Read the model definition and answer for the solid it produces. Units are mm, in the model's axes. Face numbers are marked on the shaded views. A direction names the side the tool comes from. Round coordinates to 2 decimals unless told otherwise and drop trailing zeros. Loops run counter-clockwise (first coordinate to the right, second up) from the corner with the lowest first, then second, coordinate; pieces in that order, holes last. Notation, with made-up numbers: M -3,13.5 L 40,13.5 A37 ccw 40,49.5 Z; hole C 46.25,6.25 d6. An arc over 180 degrees is marked long. Write each question's results on one line, items separated by ' | '.
Autodesk Inventor part; units mm, degrees
ref_plane "YZ Plane" through (0, 0, 0) normal (1, 0, 0) x (0, 1, 0)
ref_plane "XZ Plane" through (0, 0, 0) normal (0, 1, 0) x (-1, 0, 0)
ref_plane "XY Plane" through (0, 0, 0) normal (0, 0, 1) x (1, 0, 0)
sketch "Sketch1" plane through (0, 0, 0) normal (0, 0, 1) x (1, 0, 0)
  line L0 (-21, 8) -> (21, 8)
  line L1 (21, 8) -> (21, -21)
  line L2 (21, -21) -> (-21, -21)
  line L3 (-21, -21) -> (-21, 8)
  point P0 (0, 0)
  point P1 (0, -21)
  dimension "d0" = 21
  dimension "d1" = 42
  dimension "d2" = 29
extrude "Extrusion1" add sketch "Sketch1" along normal blind 15
fillet "Fillet1" radius 5 4 edges at (21, -21, 7.5) (-21, 8, 7.5) (21, 8, 7.5) (-21, -21, 7.5)
sketch "Sketch2" plane through (0, 0, 15) normal (0, 0, 1) x (1, 0, 0)
  line L0 (16, 8) -> (-16, 8)
  arc A0 (-11.05, 0) -> (11.05, 0) centre (0, 0) ccw
  line L1 (-11.05, 0) -> (-11.05, 8)
  line L2 (11.05, 0) -> (11.05, 8)
  dimension "d6" = 11.05
extrude "Extrusion2" cut sketch "Sketch2" against normal blind 3
sketch "Sketch3" plane through (0, 0, 12) normal (0, 0, 1) x (1, 0, 0)
  arc A0 (-11.05, 0) -> (11.05, 0) centre (0, 0) ccw
  line L0 (-11.05, 8) -> (11.05, 8)
  line L1 (-6.5, 8) -> (-6.5, 0)
  arc A1 (-6.5, 0) -> (6.5, 0) centre (0, 0) ccw
  line L2 (6.5, 0) -> (6.5, 8)
  dimension "d10" = 13
extrude "Extrusion3" cut sketch "Sketch3" against normal through all
sketch "Sketch4" plane through (-16, -21, 0) normal (0, -1, 0) x (1, 0, 0)
  line L0 (32, 0) -> (0, 0)
  line L1 (0, 15) -> (32, 15)
  line L2 (9.875, 5.5) -> (22.125, 5.5)
  circle A0 centre (9.875, 5.5) radius 1
  circle A1 centre (22.125, 5.5) radius 1
  point P0 (16, 0)
  point P1 (16, 0)
  point P2 (16, 5.5)
  dimension "d14" = 5.5
  dimension "d15" = 12.25
  dimension "d16" = 2
extrude "Extrusion4" cut sketch "Sketch4" against normal through all
sketch "Sketch5" plane through (0, 0, 0) normal (0, 0, -1) x (-1, 0, 0)
  arc A0 (-6.5, 0) -> (6.5, 0) centre (0, 0) ccw
  line L0 (-15.5, -15.5) -> (-15.5, 15.5)
  line L1 (-15.5, 15.5) -> (15.5, 15.5)
  line L2 (15.5, 15.5) -> (15.5, -15.5)
  line L3 (15.5, -15.5) -> (-15.5, -15.5)
  circle A1 centre (-15.5, -15.5) radius 1.55
  circle A2 centre (15.5, -15.5) radius 1.55
  dimension "d19" = 31
  dimension "d20" = 3.1
extrude "Extrusion5" cut sketch "Sketch5" against normal through all contours L3 A1 L0 | L0 A1 L3 | A2 L2 L3 | L3 L2 A2
properties part number "UHMW_block"
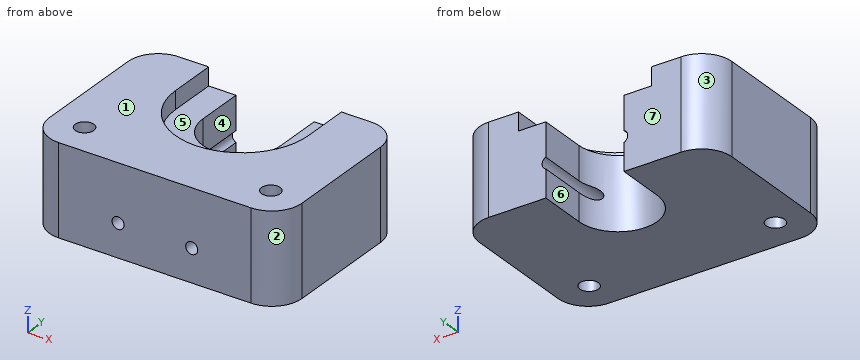
Item 1: The part is cut by section C-C (x = 15.5). Determine the outline of the cut face in (y, z), plus the area to 4 significant figures.
Outcome:
outline: M -21,0 L -17.05,0 L -17.05,15 L -21,15 Z; M -13.95,0 L 8,0 L 8,15 L -13.95,15 Z | area: 388.5 mm2
Item 2: The part is cut by section B-B (z = 8.75). Determine the outline of the cut face in (x, y), plus the area to 3 significant figures.
Outcome:
outline: M -21,-16 A5 ccw -16,-21 L 16,-21 A5 ccw 21,-16 L 21,3 A5 ccw 16,8 L 6.5,8 L 6.5,0 A6.5 cw -6.5,0 L -6.5,8 L -16,8 A5 ccw -21,3 Z; hole C -15.5,-15.5 d3.1; hole C 15.5,-15.5 d3.1 | area: 1,010 mm2
Item 3: The part is cut by section D-D (y = 5). Determine the outline of the cut face in (x, z) (3 decimals), plus the area to 4 significant figures.
Outcome:
outline: M -20.583,0 L -6.5,0 L -6.5,4.573 A1 cw -6.5,6.427 L -6.5,12 L -11.05,12 L -11.05,15 L -20.583,15 Z; M 6.5,0 L 20.583,0 L 20.583,15 L 11.05,15 L 11.05,12 L 6.5,12 L 6.5,6.427 A1 cw 6.5,4.573 Z | area: 393.5 mm2
Item 4: Flat-ended cylindrical pins translate along their axes: pin 1 (6 mm diameter, centred on y = 3.5, z = 10.5, fed in from -X); pin 2 (0.9 mm diameter, centred on y = 6, z = 14, fed in from -X); pin 3 (1.7 mm diameter, centred on y = 4, z = 9.5, fed in from +X). Find the tip coordinate at first contact, or state that the pin passes through.
Outcome:
pin 1: stops at x = -21 | pin 2: stops at x = -20.3 | pin 3: stops at x = 21
Item 5: For the marked faces 5, 6 and 7, determine the directions among +Z, -Z, +X, -X, +Y, -Y from which every point of the face is accessible in a straight line to the end or side of a thin tool.
Outcome:
face 5: +Z, +Y | face 6: +Z, -Z, +Y | face 7: +Z, -Z, +X, -X, +Y
Item 6: Straight lines are drawn through the part: line 1 (X direction, y = -8.5, z = 5.5) (3 decimals); line 2 (X direction, y = -15.5, z = 14); line 3 (X direction, y = 0.5, z = 5.5) (3 decimals). For each, find the intervals that lie inside material, in ascending order.
Outcome:
line 1: x = -21 to -7.125, -5.125 to 5.125, 7.125 to 21 | line 2: x = -21 to -17.05, -13.95 to 13.95, 17.05 to 21 | line 3: x = -21 to -7.125, 7.125 to 21
Item 7: The mould has two halves that part along X. Classify the marked faces 1, 2, 3 and 4: pulls with the +X half, pulls with the -X half, needs draft (parallel to the pull), parting line crosses it, or undercut.
Outcome:
face 1: needs draft | face 2: pulls with the +X half | face 3: pulls with the -X half | face 4: undercut
Item 8: The part is cut by section A-A (y = -15.5). Determine the outline of the cut face in (x, z) (3 decimals).
Outcome:
outline: M -21,0 L -17.05,0 L -17.05,15 L -21,15 Z; M -13.95,0 L 13.95,0 L 13.95,15 L -13.95,15 Z; M 17.05,0 L 21,0 L 21,15 L 17.05,15 Z; hole C -6.125,5.5 d2; hole C 6.125,5.5 d2
